Part model, mm, in its own coordinate system. Face numbers are marked on the shaded views. A direction names the side the tool comes from. Round coordinates to 2 decimals unless told otherwise and drop trailing zeros. Write each loop counter-clockwise with the first axis right and the second up, starting at its lowest first coordinate (ties: lowest second). Pieces come first, ordered by that corner, then holes. Notation, with made-up numbers: (75, 41.25) -> (95, 41.25) arc R36 ccw to (95, 76.25) -> close; hole circle Ø5 at (2, -34). An arc over 180 degrees is marked (long way). Return JSON: item names as keys, results as strings. Group by question number.
```python
from build123d import *

# Parameters (mm, degrees)
SKETCH1_R           = 20
SKETCH1_R_2         = 8
SKETCH1_R_3         = 50
SKETCH1_R_4         = 38
BOSS_EXTRUDE1_DEPTH = 10
SKETCH1_3_R         = 20
SKETCH1_3_R_2       = 8
BOSS_EXTRUDE2_DEPTH = 25
SKETCH1_4_R         = 50
SKETCH1_4_R_2       = 38
BOSS_EXTRUDE3_DEPTH = 60
CUT_EXTRUDE1_DEPTH  = 3


with BuildPart() as part:
    # Sketch1 → Boss-Extrude1 (new body)
    # profile 1 of 5: a face of its own
    with BuildSketch(Plane(origin=(0, 0, 0), x_dir=(1, 0, 0), z_dir=(0, 1, 0))):
        with BuildLine():
            ThreePointArc((-15, -47.696960071), (-50, 0), (-15, 47.696960071))
            Line((-15, 47.696960071), (-106, 19.078784028))
            ThreePointArc((-106, 19.078784028), (-88.167840434, 16.124515497), (-80, 0))
            ThreePointArc((-80, 0), (-88.167840434, -16.124515497), (-106, -19.078784028))
            Line((-106, -19.078784028), (-15, -47.696960071))
        make_face()
    # profile 2 of 5: a face of its own
    with BuildSketch(Plane(origin=(0, 0, 0), x_dir=(1, 0, 0), z_dir=(0, 1, 0))):
        with Locations((-100, 0)):
            Circle(SKETCH1_R)
        with Locations(Location((-100, 0, 0), (0, 0, 270))):
            Circle(SKETCH1_R_2, mode=Mode.SUBTRACT)
    # profile 3 of 5: a face of its own
    with BuildSketch(Plane(origin=(0, 0, 0), x_dir=(1, 0, 0), z_dir=(0, 1, 0))):
        Circle(SKETCH1_R_3)
        with Locations(Location((0, 0, 0), (0, 0, 270))):
            Circle(SKETCH1_R_4, mode=Mode.SUBTRACT)
    # profile 4 of 5: a face of its own
    with BuildSketch(Plane(origin=(0, 0, 0), x_dir=(1, 0, 0), z_dir=(0, 1, 0))):
        with BuildLine():
            Line((106, 19.078784028), (15, 47.696960071))
            ThreePointArc((15, 47.696960071), (40.311288741, 29.580398915), (50, 0))
            ThreePointArc((50, 0), (40.311288741, -29.580398915), (15, -47.696960071))
            Line((15, -47.696960071), (106, -19.078784028))
            ThreePointArc((106, -19.078784028), (80, 0), (106, 19.078784028))
        make_face()
    # profile 5 of 5: a face of its own
    with BuildSketch(Plane(origin=(0, 0, 0), x_dir=(1, 0, 0), z_dir=(0, 1, 0))):
        with Locations((100, 0)):
            Circle(SKETCH1_R)
        with Locations(Location((100, 0, 0), (0, 0, 270))):
            Circle(SKETCH1_R_2, mode=Mode.SUBTRACT)
    extrude(amount=BOSS_EXTRUDE1_DEPTH)

    # Sketch1_3 → Boss-Extrude2 (add)
    # profile 1 of 2: a face of its own
    with BuildSketch(Plane(origin=(0, 0, 0), x_dir=(1, 0, 0), z_dir=(0, 1, 0))):
        with Locations(Location((-100, 0, 0), (0, 0, 107.457603124))):
            Circle(SKETCH1_3_R)
        with Locations(Location((-100, 0, 0), (0, 0, 270))):
            Circle(SKETCH1_3_R_2, mode=Mode.SUBTRACT)
    # profile 2 of 2: a face of its own
    with BuildSketch(Plane(origin=(0, 0, 0), x_dir=(1, 0, 0), z_dir=(0, 1, 0))):
        with Locations(Location((100, 0, 0), (0, 0, 72.542396876))):
            Circle(SKETCH1_3_R)
        with Locations(Location((100, 0, 0), (0, 0, 270))):
            Circle(SKETCH1_3_R_2, mode=Mode.SUBTRACT)
    extrude(amount=BOSS_EXTRUDE2_DEPTH)

    # Sketch1_4 → Boss-Extrude3 (add)
    with BuildSketch(Plane(origin=(0, 0, 0), x_dir=(1, 0, 0), z_dir=(0, 1, 0))):
        with Locations(Location((0, 0, 0), (0, 0, 107.457603124))):
            Circle(SKETCH1_4_R)
        with Locations(Location((0, 0, 0), (0, 0, 270))):
            Circle(SKETCH1_4_R_2, mode=Mode.SUBTRACT)
    extrude(amount=BOSS_EXTRUDE3_DEPTH)

    # Sketch5 → Cut-Extrude1 (cut)
    with BuildSketch(Plane(origin=(0, 10, 0), x_dir=(1, 0, 0), z_dir=(0, 1, 0))):
        with BuildLine():
            Line((-33.478784028, -39.789081668), (-93.333517497, -20.965638818))
            ThreePointArc((-93.333517497, -20.965638818), (-78, 0), (-93.333517497, 20.965638818))
            Line((-93.333517497, 20.965638818), (-33.478784028, 39.789081668))
            ThreePointArc((-33.478784028, 39.789081668), (-52, 0), (-33.478784028, -39.789081668))
        make_face()
        with BuildLine():
            Line((93.333517497, 20.965638818), (33.478784028, 39.789081668))
            ThreePointArc((33.478784028, 39.789081668), (52, 0), (33.478784028, -39.789081668))
            Line((33.478784028, -39.789081668), (93.333517497, -20.965638818))
            ThreePointArc((93.333517497, -20.965638818), (78, 0), (93.333517497, 20.965638818))
        make_face()
    extrude(amount=-CUT_EXTRUDE1_DEPTH, mode=Mode.SUBTRACT)


solid = part.part
```
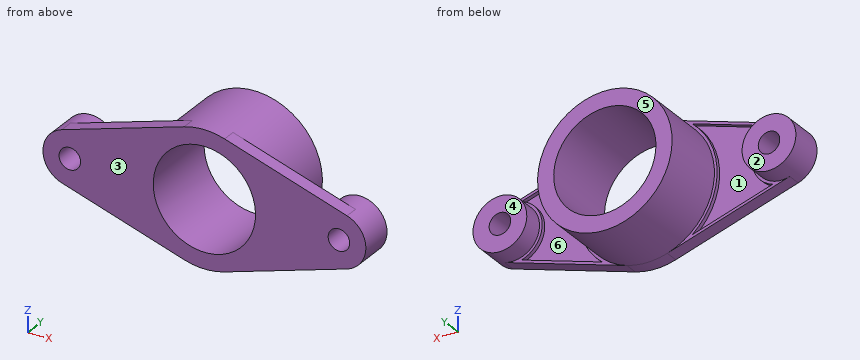
Item 1: Which spindle directions (+Z, -Z, +X, -X, +Y, -Y) get a long thin tool onto all of the face, cutting with end or side? Do the marked faces 1, 2, 3 and 4. Say none if no direction does.
Item 2: Cut at C-C (z = 0). State how many separate pieces and enclosed holes the cut face has, then the cut area to 3 significant figures.
Item 3: Flat gauge pins, fed straight in: P1, Ø12, axis at y = 47.5, z = 9.5, coming from the +X side; P2, Ø4, axis at x = -23.5, y = 30.5, coming from the +Z side; P3, Ø3, axis at x = -91, z = -9.5, coming from the +Y side; P4, Ø13, axis at x = -100, z = 0, coming from the +Y side. Where does each tip first touch, or does it go through?
Item 4: Cut at D-D (x = -100). Write the cut outline in (y, z), then the cut area to 3 significant figures.
Item 5: Cut at A-A (x = 0). Write the cut outline in (y, z).
Item 6: Wall check: L1, parallel to X at y = 15, z = 0; L2, parallel to X at y = 6.5, z = 0; L3, parallel to X at y = 39, z = 0. Give the ranges that are in metal, low to high.
Item 7: Two-plate mould, pull along X, no slides. Class the marked faces 5 and 6: released by +X, released by -X, zero draft, split by the parting line, or undercut.
Item 8: Cut at B-B (y = 20). Write the cut outline in (x, z).
Checks:
{
 "1": {"face 1": "+Y", "face 2": "+Z, -Z, -X, +Y", "face 3": "+Z, -Z, +X, -X, -Y", "face 4": "+Z, -Z, +X, +Y"},
 "2": {"separate pieces": "4", "enclosed holes": "0", "area": "3,080 mm2"},
 "3": {"P1": "stops at x = 49.88", "P2": "stops at z = 45.14", "P3": "stops at y = 25", "P4": "passes through"},
 "4": {"outline": "(0, -20.97) -> (10, -20.97) -> (10, -20) -> (25, -20) -> (25, -8) -> (0, -8) -> close; (0, 8) -> (25, 8) -> (25, 20) -> (10, 20) -> (10, 20.97) -> (0, 20.97) -> close", "area": "619 mm2"},
 "5": {"outline": "(0, -50) -> (60, -50) -> (60, -38) -> (0, -38) -> close; (0, 38) -> (60, 38) -> (60, 50) -> (0, 50) -> close"},
 "6": {"L1": "x = -120 to -108, -92 to -80, -50 to -38, 38 to 50, 80 to 92, 108 to 120", "L2": "x = -120 to -108, -92 to -38, 38 to 92, 108 to 120", "L3": "x = -50 to -38, 38 to 50"},
 "7": {"face 5": "zero draft", "face 6": "undercut"},
 "8": {"outline": "circle Ø40 at (-100, 0); circle Ø100 at (0, 0); circle Ø40 at (100, 0); hole circle Ø16 at (-100, 0); hole circle Ø76 at (0, 0); hole circle Ø16 at (100, 0)"}
}
